Study the drawing (mm; zero at the part's minimum x, y, z) and answer. A direction names the side the tool comes from. Give positions to 0.01 mm unless a question says otherwise; leave off trailing zeros. Write each loop counter-clockwise with the first axis right and the second up, starting at its lowest first coordinate (ties: lowest second). Pieces come first, ordered by that corner, then holes. Notation, with made-up numbers: (-10.75, -17.75) - (18.25, -17.75) arc R10 ccw to (18.25, -0.75) - close; hole circle Ø9 at (-6, 35.25). An arc over 180 degrees is marked (long way). Write each question's results on one line, items separated by ' | '. Start each with the question number.
Q1. For the marked faces 1 and 2, determine the directions among +Z, -Z, +X, -X, +Y, -Y from which every point of the face is accessible in a straight line to the end or side of a thin tool.
Q2. Section C-C (y = 11.5) is taken. Determine the outline of the cut face in (x, z), plus the area to 3 significant figures.
Q3. For a pull along X with two mould halves and no side action, classify the marked faces 3, 4 and 5 as pulls with the +X half, pulls with the -X half, needs draft (parallel to the pull), parting line crosses it, or undercut.
Q4. Section D-D (z = 50) is taken. Determine the outline of the cut face in (x, y).
Q5. Section A-A (y = 50) is taken. Determine the outline of the cut face in (x, z) (1 decimal).
Q6. Flat-ended cylindrical pins translate along their axes: pin 1 Ø13 at (x, y) = (91.5, 91.5) entering from +Z; pin 2 Ø6.5 at (y, z) = (9, 58.5) entering from -X; pin 3 Ø4 at (x, y) = (26, 43.5) entering from -Z (1 decimal); pin 4 Ø6 at (x, z) = (58.5, 60) entering from -Y. Find the tip coordinate at first contact, or state that the pin passes through.
Q7. Section B-B (x = 90) is taken. Determine the outline of the cut face in (y, z) (1 decimal).
Q8. Find the intervals of material crossed by probe 1 along Y at (x, z) = (90, 31); probe 2 along X at (y, z) = (50, 47) (1 decimal); probe 3 along X at (y, z) = (50, 51.5) (1 decimal), in increasing order.
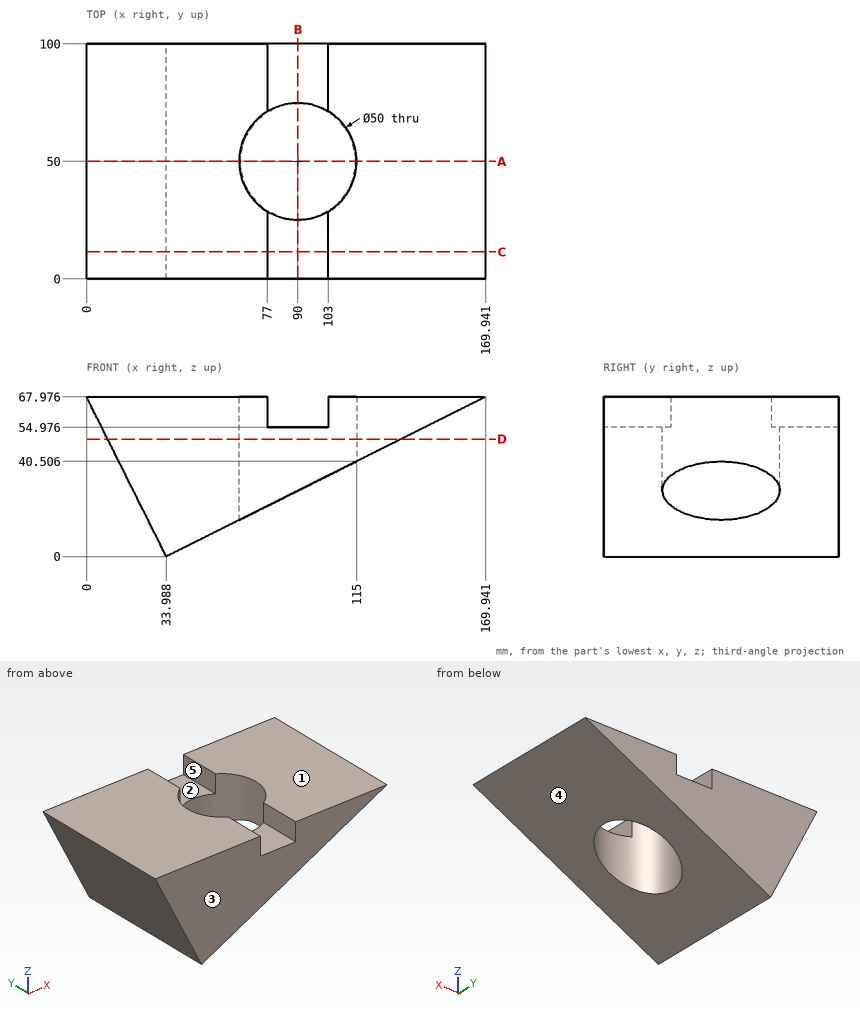
Answers below:
1) face 1: +Z, +X, -X, +Y, -Y | face 2: +Z, +Y, -Y
2) outline: (0, 67.98) - (33.99, 0) - (169.94, 67.98) - (103, 67.98) - (103, 54.98) - (77, 54.98) - (77, 67.98) - close | area: 5,440 mm2
3) face 3: needs draft | face 4: pulls with the +X half | face 5: undercut
4) outline: (8.99, 0) - (133.99, 0) - (133.99, 100) - (8.99, 100) - close; hole circle Ø50 at (90, 50)
5) outline: (0, 68) - (34, 0) - (65, 15.5) - (65, 68) - close; (115, 40.5) - (169.9, 68) - (115, 68) - close
6) pin 1: stops at z = 54.98 | pin 2: stops at x = 3.11 | pin 3: stops at z = 12 | pin 4: stops at y = 0
7) outline: (0, 28) - (25, 28) - (25, 55) - (0, 55) - close; (75, 28) - (100, 28) - (100, 55) - (75, 55) - close
8) probe 1: y = 0 to 25, 75 to 100 | probe 2: x = 10.5 to 65, 115 to 128 | probe 3: x = 8.2 to 65, 115 to 137
